from build123d import *

# Parameters (mm, degrees)
BASE_DEPTH                  = 3
CROQUIS2_W                  = 50
CROQUIS2_H                  = 28.1
SALIENTE_EXTRUIR2_DEPTH     = 15.5
CORTAR_EXTRUIR1_REACH       = 92.946
CORTAR_EXTRUIR2_REACH       = 88.329
CROQUIS15_W                 = 100
CROQUIS15_H                 = 54.46
SALIENTE_EXTRUIR3_DEPTH     = 3.6
CORTAR_EXTRUIR3_DEPTH       = 3.6
CROQUIS5_R                  = 1.2
CORTAR_EXTRUIR4_DEPTH       = 6
CORTAR_EXTRUIR7_DEPTH       = 113.455546773
SALIENTE_EXTRUIR5_DEPTH     = 100
CHAFL_N1_SIZE               = 3
CORTAR_EXTRUIR9_DEPTH       = 25
CORTAR_EXTRUIR10_START      = -25
CORTAR_EXTRUIR10_DEPTH      = 25
CORTAR_EXTRUIR11_DEPTH      = 18
CORTAR_EXTRUIR14_DEPTH      = 10
CORTAR_EXTRUIR14_DEPTH_BACK = 10
CROQUIS45_W                 = 12.1
CROQUIS45_H                 = 9.1
CORTAR_EXTRUIR15_DEPTH      = 10
CORTAR_EXTRUIR15_DEPTH_BACK = 10
CROQUIS49_W                 = 12.1
CROQUIS49_H                 = 9.1
CROQUIS63_W                 = 12.1
CROQUIS63_H                 = 9.1
CORTAR_EXTRUIR19_DEPTH      = 30
CROQUIS64_W                 = 9.1
CROQUIS64_H                 = 12.1
CORTAR_EXTRUIR20_DEPTH      = 10
CROQUIS66_W                 = 9.1
CROQUIS66_H                 = 12.1
CORTAR_EXTRUIR21_DEPTH      = 10
SALIENTE_EXTRUIR11_DEPTH    = 18
CROQUIS73_R                 = 1.7
CORTAR_EXTRUIR22_DEPTH      = 10
CROQUIS75_W                 = 13.5
CROQUIS75_H                 = 7.5
CORTAR_EXTRUIR26_DEPTH      = 1
CORTAR_EXTRUIR27_DEPTH      = 76.642628391


with BuildPart() as part:
    # Croquis1 → Base (new body)
    with BuildSketch(Plane.XY):
        Polygon((-50, -48), (50, -48), (50, 19.9), (25, 19.9), (25, 48), (-25, 48), (-25, 19.9), (-50, 19.9), align=None)
    extrude(amount=BASE_DEPTH)

    # Croquis2 → Saliente-Extruir2 (add)
    with BuildSketch(Plane.XY.offset(3)):
        with Locations((0, 33.95)):
            Rectangle(CROQUIS2_W, CROQUIS2_H)
    extrude(amount=SALIENTE_EXTRUIR2_DEPTH)

    # Croquis3 → Cortar-Extruir1 (cut, up to next)
    with BuildSketch(Plane.ZY.offset(25), mode=Mode.PRIVATE) as cortar_extruir1_sk1:
        with BuildLine():
            Line((18.5, 40), (18.5, 27.9))
            Line((18.5, 27.9), (9, 27.9))
            ThreePointArc((9, 27.9), (5.931506818, 33.95), (9, 40))
            Line((9, 40), (18.5, 40))
        make_face()
    cortar_extruir1_tool1 = extrude(cortar_extruir1_sk1.sketch, amount=-CORTAR_EXTRUIR1_REACH, mode=Mode.PRIVATE) & part.part
    add(cortar_extruir1_tool1.solids().sort_by_distance((-25, 33.95, 12.643483))[0], mode=Mode.SUBTRACT)

    # Croquis4 → Cortar-Extruir2 (cut, up to next)
    with BuildSketch(Plane.XZ.offset(-19.9), mode=Mode.PRIVATE) as cortar_extruir2_sk1:
        with BuildLine():
            Line((1, 15.5), (-1, 15.5))
            ThreePointArc((-1, 15.5), (-3.121320344, 16.378679656), (-4, 18.5))
            Line((-4, 18.5), (4, 18.5))
            ThreePointArc((4, 18.5), (3.121320344, 16.378679656), (1, 15.5))
        make_face()
    cortar_extruir2_tool1 = extrude(cortar_extruir2_sk1.sketch, amount=-CORTAR_EXTRUIR2_REACH, mode=Mode.PRIVATE) & part.part
    add(cortar_extruir2_tool1.solids().sort_by_distance((0, 19.9, 17.159196))[0], mode=Mode.SUBTRACT)

    # Croquis15 → Saliente-Extruir3 (add)
    with BuildSketch(Plane.XY.offset(3)):
        with Locations((0, -7.33)):
            Rectangle(CROQUIS15_W, CROQUIS15_H)
    extrude(amount=SALIENTE_EXTRUIR3_DEPTH)

    # Croquis16 → Cortar-Extruir3 (cut)
    with BuildSketch(Plane(origin=(0, 0, 0), x_dir=(-1, 0, 0), z_dir=(0, 0, -1))):
        Polygon((25, 19.9), (50, 19.9), (50, -48), (-50, -48), (-50, 19.9), (-25, 19.9), align=None)
    extrude(amount=-CORTAR_EXTRUIR3_DEPTH, mode=Mode.SUBTRACT)

    # Croquis5 → Cortar-Extruir4 (cut)
    with BuildSketch(Plane.XY.offset(18.5)):
        with Locations((-20, 44)):
            Circle(CROQUIS5_R)
        with Locations((-8, 44)):
            Circle(CROQUIS5_R)
        with Locations((-20, 23.9)):
            Circle(CROQUIS5_R)
        with Locations((-8, 23.9)):
            Circle(CROQUIS5_R)
        with Locations((8, 44)):
            Circle(CROQUIS5_R)
        with Locations((20, 44)):
            Circle(CROQUIS5_R)
        with Locations((8, 23.9)):
            Circle(CROQUIS5_R)
        with Locations((20, 23.9)):
            Circle(CROQUIS5_R)
    extrude(amount=-CORTAR_EXTRUIR4_DEPTH, mode=Mode.SUBTRACT)

    # Croquis22 → Cortar-Extruir7 (cut, through all)
    with BuildSketch(Plane.ZY.offset(50)):
        Polygon((4.66, -30.6), (6.6, -29.479940478), (6.6, -34.56), (3.6, -34.56), align=None)
    extrude(amount=-CORTAR_EXTRUIR7_DEPTH, mode=Mode.SUBTRACT)

    # Croquis24 → Saliente-Extruir5 (add, through all)
    with BuildSketch(Plane.ZY.offset(50)):
        with BuildLine():
            Line((24.6, -14.479940478), (40.345333467, -14.479940478))
            Line((40.345333467, -14.479940478), (40.345333467, -16.479940478))
            ThreePointArc((40.345333467, -16.479940478), (22.538840373, -20.555918791), (6.6, -29.479940478))
            Line((6.6, -29.479940478), (6.6, 19.9))
            Line((6.6, 19.9), (24.6, 19.9))
            Line((24.6, 19.9), (24.6, -14.479940478))
        make_face()
    extrude(amount=-SALIENTE_EXTRUIR5_DEPTH)

    # Chaflán1
    chafl_n1_edges = [part.edges().sort_by_distance(p)[0] for p in [
        (0, 48, 0),
    ]]
    chamfer(chafl_n1_edges, length=CHAFL_N1_SIZE)

    # Croquis25 → Cortar-Extruir9 (cut)
    with BuildSketch(Plane.ZY.offset(50)):
        with BuildLine():
            Line((23.26, 19.9), (3.6, 19.9))
            ThreePointArc((3.6, 19.9), (13.43, 16.802656182), (23.26, 19.9))
        make_face()
    extrude(amount=-CORTAR_EXTRUIR9_DEPTH, mode=Mode.SUBTRACT)

    # Croquis26 → Cortar-Extruir10 (cut)
    with BuildSketch(Plane(origin=(50, 0, 0), x_dir=(0, 0, -1), z_dir=(1, 0, 0)).offset(CORTAR_EXTRUIR10_START)):
        with BuildLine():
            Line((-3.6, 19.9), (-23.26, 19.9))
            ThreePointArc((-23.26, 19.9), (-13.43, 16.802656182), (-3.6, 19.9))
        make_face()
    extrude(amount=CORTAR_EXTRUIR10_DEPTH, mode=Mode.SUBTRACT)

    # Croquis28 → Cortar-Extruir11 (cut)
    with BuildSketch(Plane.XY.offset(24.6)):
        Polygon((-43, -9.479940478), (-43, 19.9), (43, 19.9), (43, -9.479940478), (43, -14.479940478), (-43, -14.479940478), align=None)
    extrude(amount=-CORTAR_EXTRUIR11_DEPTH, mode=Mode.SUBTRACT)

    # Croquis45 → Cortar-Extruir14 (cut, two sides: drawn at the far end of the back side and taken through both)
    with BuildSketch(Plane(origin=(-7.65, -28.550188678, 0), x_dir=(-0.9659258262890681, 0.25881904510252135, 0), z_dir=(-0.25881904510252135, -0.9659258262890681, 0)).offset(-CORTAR_EXTRUIR14_DEPTH_BACK)):
        with Locations((22.96204173, -14.6)):
            Rectangle(CROQUIS45_W, CROQUIS45_H)
    extrude(amount=CORTAR_EXTRUIR14_DEPTH + CORTAR_EXTRUIR14_DEPTH_BACK, mode=Mode.SUBTRACT)

    # Croquis49 → Cortar-Extruir15 (cut, two sides: drawn at the far end of the back side and taken through both)
    with BuildSketch(Plane(origin=(7.65, -28.550188678, 0), x_dir=(-0.96592582628907, -0.2588190451025146, 0), z_dir=(0.2588190451025145, -0.9659258262890699, 0)).offset(-CORTAR_EXTRUIR15_DEPTH_BACK)):
        with Locations((-22.96204173, -14.6)):
            Rectangle(CROQUIS49_W, CROQUIS49_H)
    extrude(amount=CORTAR_EXTRUIR15_DEPTH + CORTAR_EXTRUIR15_DEPTH_BACK, mode=Mode.SUBTRACT)

    # Croquis63 → Cortar-Extruir19 (cut)
    with BuildSketch(Plane(origin=(0, -14.479940478, 0), x_dir=(1, 0, 0), z_dir=(0, 1, 0))):
        with Locations((0.063130338, -14.6)):
            Rectangle(CROQUIS63_W, CROQUIS63_H)
    extrude(amount=-CORTAR_EXTRUIR19_DEPTH, mode=Mode.SUBTRACT)

    # Croquis64 → Cortar-Extruir20 (cut)
    with BuildSketch(Plane.ZY.offset(50)):
        with Locations((8.15, -3.1)):
            Rectangle(CROQUIS64_W, CROQUIS64_H)
    extrude(amount=-CORTAR_EXTRUIR20_DEPTH, mode=Mode.SUBTRACT)

    # Croquis66 → Cortar-Extruir21 (cut)
    with BuildSketch(Plane(origin=(50, 0, 0), x_dir=(0, 0, -1), z_dir=(1, 0, 0))):
        with Locations((-8.15, -3.1)):
            Rectangle(CROQUIS66_W, CROQUIS66_H)
    extrude(amount=-CORTAR_EXTRUIR21_DEPTH, mode=Mode.SUBTRACT)

    # Croquis70 → Saliente-Extruir11 (add)
    with BuildSketch(Plane.XY.offset(6.6)):
        with BuildLine():
            Line((-43, -9.15), (-43, -14.479940478))
            Line((-43, -14.479940478), (-37.670059522, -14.479940478))
            ThreePointArc((-37.670059522, -14.479940478), (-41.438896577, -12.918837055), (-43, -9.15))
        make_face()
        with BuildLine():
            Line((43, -14.479940478), (43, -9.15))
            ThreePointArc((43, -9.15), (41.438896577, -12.918837055), (37.670059522, -14.479940478))
            Line((37.670059522, -14.479940478), (43, -14.479940478))
        make_face()
    extrude(amount=SALIENTE_EXTRUIR11_DEPTH)

    # Croquis73 → Cortar-Extruir22 (cut)
    with BuildSketch(Plane(origin=(0, 0, 3.6), x_dir=(-1, 0, 0), z_dir=(0, 0, -1))):
        with Locations((-45, 11.425)):
            Circle(CROQUIS73_R)
        with Locations((45, 11.425)):
            Circle(CROQUIS73_R)
        with Locations((45, -20.575)):
            Circle(CROQUIS73_R)
        with Locations((-45, -20.575)):
            Circle(CROQUIS73_R)
    extrude(amount=-CORTAR_EXTRUIR22_DEPTH, mode=Mode.SUBTRACT)

    # Croquis75 → Cortar-Extruir26 (cut)
    with BuildSketch(Plane(origin=(0, 0, 3.6), x_dir=(-1, 0, 0), z_dir=(0, 0, -1))):
        with Locations((-35, -30.81)):
            Rectangle(CROQUIS75_W, CROQUIS75_H)
        with Locations((35, -30.81)):
            Rectangle(CROQUIS75_W, CROQUIS75_H)
    extrude(amount=-CORTAR_EXTRUIR26_DEPTH, mode=Mode.SUBTRACT)

    # Croquis76 → Cortar-Extruir27 (cut, through all)
    with BuildSketch(Plane.XY.offset(10.05)):
        Polygon((-29.251017738, -34.56), (-36.815799839, -34.56), (-31.435364106, -14.479940478), (-23.870582005, -14.479940478), align=None)
        Polygon((29.251017738, -34.56), (23.870582005, -14.479940478), (31.435364106, -14.479940478), (36.815799839, -34.56), align=None)
    extrude(amount=-CORTAR_EXTRUIR27_DEPTH, mode=Mode.SUBTRACT)


solid = part.part
For this review, take the finished solid that the model builds, in its own axes (mm). A direction names the side the tool comes from. Coordinates: 2 decimals unless noted, no trailing zeros. Loops run counter-clockwise (first coordinate to the right, second up) from the corner with the lowest first, then second, coordinate; pieces in that order, holes last. Notation, with made-up numbers: (30, 0) - (68, 0) arc R20 cw to (68, 25) - close; hole circle Ø2 at (54.5, 89). An arc over 180 degrees is marked (long way). Return JSON: item names as keys, results as strings.
Item 1: Take a section at C-C (y = 23.9). Give the boundary of the cut face in (x, z), then the cut area to 3 significant figures.
Determined:
{"outline": "(-25, 0) - (25, 0) - (25, 18.5) - (21.2, 18.5) - (21.2, 12.5) - (18.8, 12.5) - (18.8, 18.5) - (9.2, 18.5) - (9.2, 12.5) - (6.8, 12.5) - (6.8, 18.5) - (4, 18.5) arc R3 cw to (1, 15.5) - (-1, 15.5) arc R3 cw to (-4, 18.5) - (-6.8, 18.5) - (-6.8, 12.5) - (-9.2, 12.5) - (-9.2, 18.5) - (-18.8, 18.5) - (-18.8, 12.5) - (-21.2, 12.5) - (-21.2, 18.5) - (-25, 18.5) - close", "area": "847 mm2"}
Item 2: For faces 4 (the flat face through (33.1, -20.7, 6.9)), 5 (the flat face through (-40, -3, 5)), 6 (the flat face through (8, 24, 12.5)), list the 3-axis set-ups (+Z, -Z, +X, -X, +Y, -Y) from which the entire face can be reached by the end or side of a thin tool; tool diameter is ignored.
Determined:
{"face 4": "-Z, -Y", "face 5": "+Z, -Z, -X", "face 6": "+Z"}
Item 3: Take a section at A-A (y = -5.5). Give the boundary of the cut face in (x, z), then the cut area to 3 significant figures.
Determined:
{"outline": "(-50, 12.7) - (-43, 12.7) - (-43, 24.6) - (-50, 24.6) - close; (-40, 3.6) - (40, 3.6) - (40, 6.6) - (-40, 6.6) - close; (43, 12.7) - (50, 12.7) - (50, 24.6) - (43, 24.6) - close", "area": "407 mm2"}
Item 4: Take a section at D-D (y = -25). Give the boundary of the cut face in (x, z), then the cut area to 3 significant figures.
Determined:
{"outline": "(-50, 3.6) - (-34.25, 3.6) - (-34.25, 10.05) - (-36.73, 10.05) - (-36.73, 13.29) - (-50, 13.29) - close; (-26.69, 3.6) - (26.69, 3.6) - (26.69, 10.05) - (24.21, 10.05) - (24.21, 13.29) - (6.11, 13.29) - (6.11, 10.05) - (-5.99, 10.05) - (-5.99, 13.29) - (-24.21, 13.29) - (-24.21, 10.05) - (-26.69, 10.05) - close; (34.25, 3.6) - (50, 3.6) - (50, 13.29) - (36.73, 13.29) - (36.73, 10.05) - (34.25, 10.05) - close", "area": "751 mm2"}
Item 5: Mouldability with a two-part tool opening along X and no side actions: class faces 1 (the cylindrical face through (7.84, 45.19, 15.54)), 2 (the flat face through (-25, 33, 5)), 3 (the flat face through (46, -9.15, 8)) as pulls with the +X half, pulls with the -X half, needs draft (parallel to the pull), parting line crosses it, or undercut.
Determined:
{"face 1": "undercut", "face 2": "pulls with the -X half", "face 3": "needs draft"}
Item 6: For line 1 (Y direction, x = -20, z = 13.7); line 2 (Y direction, x = -8, z = 14); line 3 (X direction, y = 23, z = 14), list the stretches that pass through material, from the lowest coordinate up.
Determined:
{"line 1": "y = -24.76 to -14.48, 19.9 to 22.7, 25.1 to 27.9, 40 to 42.8, 45.2 to 48", "line 2": "y = -24.59 to -14.48, 19.9 to 22.7, 25.1 to 27.9, 40 to 42.8, 45.2 to 48", "line 3": "x = -25 to -20.79, -19.21 to -8.79, -7.21 to 7.21, 8.79 to 19.21, 20.79 to 25"}
Item 7: Take a section at B-B (x = 12.5). Give the boundary of the cut face in (y, z), then the cut area to 3 significant figures.
Determined:
{"outline": "(-34.56, 3.6) - (19.9, 3.6) - (19.9, 0) - (45, 0) - (48, 3) - (48, 18.5) - (40, 18.5) - (40, 9) arc R7.5 cw to (27.9, 9) - (27.9, 18.5) - (19.9, 18.5) - (19.9, 6.6) - (-14.48, 6.6) - (-14.48, 40.35) - (-16.48, 40.35) arc R64.23 cw to (-29.48, 6.6) - (-30.6, 4.66) - close", "area": "751 mm2"}
Item 8: Insertion check: pin 1 (1 mm diameter, centred on x = -23, z = 21.5, fed in from +Y); pin 2 (1.1 mm diameter, centred on x = 3, z = 1, fed in from -Y); pin 3 (10 mm diameter, centred on x = -30.5, y = 22.5, fed in from -Z); pin 4 (20.5 mm diameter, centred on y = 26, z = 5.5, fed in from +X). Each pin has a flat end and moves straight along its axis. Give the tip position at first contact, or say it passes through.
Determined:
{"pin 1": "stops at y = -14.48", "pin 2": "stops at y = 19.9", "pin 3": "stops at z = 3.6", "pin 4": "stops at x = 50"}
